Could you check a few things on this model? Use its own coordinates, in mm. Face numbers are marked on the shaded views. A direction names the side the tool comes from. Give positions to 0.01 mm unless a question says otherwise; leave off trailing zeros. Write each loop counter-clockwise with the first axis right and the second up, starting at its lowest first coordinate (ties: lowest second). Pieces come first, ordered by that corner, then holes. Notation, with made-up numbers: M 20.25,-4.5 L 58.25,-4.5 A16 cw 58.25,14.5 Z; hole C 44.25,-12.5 d8. An arc over 180 degrees is marked long. One line per item, written item: value.
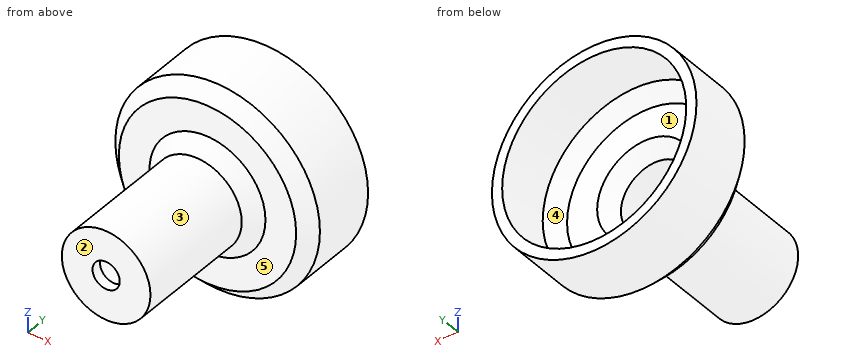
```python
from build123d import *

# Parameters (mm, degrees)
SKETCH_2_R          = 2
CUT_EXTRUDE_1_DEPTH = 1.5


with BuildPart() as part:
    # 草图1 → 旋转3 (revolve)
    with BuildSketch(Plane.XY):
        Polygon((0, 0), (5, 0), (5, 18), (7, 20), (11.418621451, 20), (13.5, 22), (13.5, 30), (15, 30), (15, 20.5), (13, 18.5), (8.5, 18.5), (6.5, 16.5), (6.5, -1.5), (5, -1.5), (0, -1.5), align=None)
    revolve(axis=Axis((0, -297.326720661, 0), (0, 1, 0)))

    # 草图2 → 切除-拉伸1 (cut)
    with BuildSketch(Plane(origin=(0, 0, 0), x_dir=(1, 0, 0), z_dir=(0, 1, 0))):
        with Locations(Location((0, 0, 0), (0, 0, 180))):
            Circle(SKETCH_2_R)
    extrude(amount=-CUT_EXTRUDE_1_DEPTH, mode=Mode.SUBTRACT)


solid = part.part
```
1) I'm going to push flat-ended pins straight in: pin 1 (7 mm diameter, centred on x = -4.5, z = -2.5, fed in from +Y); pin 2 (1 mm diameter, centred on x = 9.5, z = 2, fed in from -Y); pin 3 (1.5 mm diameter, centred on x = -3, z = 0.5, fed in from +Y). Where does each tip first touch, or does it pass through?
Outcome:
pin 1: stops at y = 20
pin 2: stops at y = 18.5
pin 3: stops at y = 0
2) If we section it at A-A, the plane z = 0: Write out the boundary of the cut face in (x, y).
Outcome:
outline: M -15,20.5 L -13,18.5 L -8.5,18.5 L -6.5,16.5 L -6.5,-1.5 L -2,-1.5 L -2,0 L -5,0 L -5,18 L -7,20 L -11.42,20 L -13.5,22 L -13.5,30 L -15,30 Z; M 2,-1.5 L 6.5,-1.5 L 6.5,16.5 L 8.5,18.5 L 13,18.5 L 15,20.5 L 15,30 L 13.5,30 L 13.5,22 L 11.42,20 L 7,20 L 5,18 L 5,0 L 2,0 Z
3) If we section it at B-B, the plane x = 0: Write out the boundary of the cut face in (y, z), then the cut area to 3 significant figures.
Outcome:
outline: M -1.5,-6.5 L 16.5,-6.5 L 18.5,-8.5 L 18.5,-13 L 20.5,-15 L 30,-15 L 30,-13.5 L 22,-13.5 L 20,-11.42 L 20,-7 L 18,-5 L 0,-5 L 0,-2 L -1.5,-2 Z; M -1.5,2 L 0,2 L 0,5 L 18,5 L 20,7 L 20,11.42 L 22,13.5 L 30,13.5 L 30,15 L 20.5,15 L 18.5,13 L 18.5,8.5 L 16.5,6.5 L -1.5,6.5 Z
area: 129 mm^2
4) On a 3-axis mill with a long thin cutter (end or side, diameter ignored), from which of +Z, -Z, +X, -X, +Y, -Y can I reach the whole of each face in a straight line? I mean the marked faces 1 and 2. Say none if no direction works.
Outcome:
face 1: +Y
face 2: +Z, -Z, +X, -X, -Y
5) We'd pull the mould along X, two halves only. Please class the marked faces 3, 4 and 5: pulls with the +X half, pulls with the -X half, needs draft (parallel to the pull), parting line crosses it, or undercut.
Outcome:
face 3: parting line crosses it
face 4: undercut
face 5: needs draft
6) If we section it at C-C, the plane y = 15.5: Write out the boundary of the cut face in (x, z).
Outcome:
outline: C 0,0 d13; hole C 0,0 d10
7) Please list where these lines run through material, in increasing order: L1, parallel to Z at x = 0, y = 10.5; L2, parallel to Z at x = 0, y = -1.1. Write a range as from..to.
Outcome:
L1: z = -6.5..-5, 5..6.5
L2: z = -6.5..-2, 2..6.5
